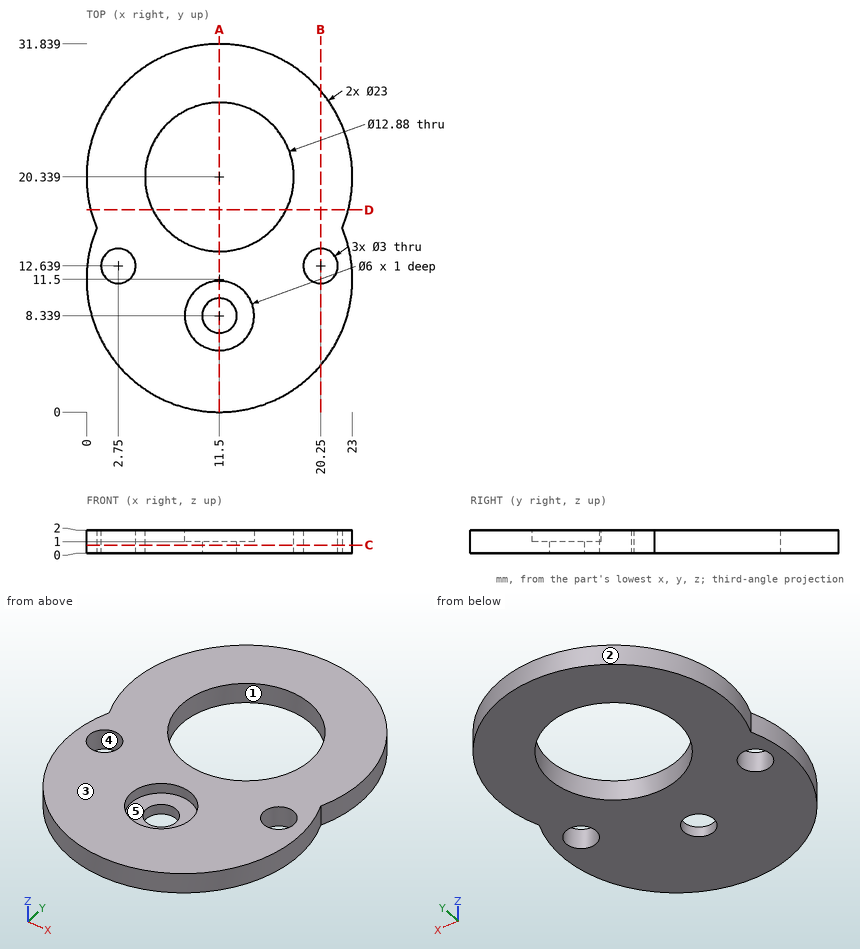
Could you check a few things on this drawing? It's one solid part, dimensions in mm from its lowest x, y, z. A direction names the side the tool comes from. Coordinates: 2 decimals unless noted, no trailing zeros. Order: outer loops, then holes, each group sorted by start corner. A loop starts at its lowest first (then second) coordinate and runs counter-clockwise, first axis right, second up. Notation, with made-up numbers: (50, 59) -> (58, 59) arc R34 ccw to (58, 89) -> close; hole circle Ø6 at (-33, -32.5). An arc over 180 degrees is marked (long way). Answer in a Markdown table with one row per item.
(1) Thinking about a two-plate mould opening in X: for the marked faces 1, 2 and 3, which applies, +X half, -X half, draft (parallel to the pull), parting line (faces both ways), or undercut?
Answer key:
| item | result |
|---|---|
| face 1 | undercut |
| face 2 | parting line |
| face 3 | draft |
(2) Will this pin go through, and if not, where does the flat tip stop? pin 1 Ø1.8 at (x, y) = (10.5, 8) entering from +Z.
Answer key:
| item | result |
|---|---|
| pin 1 | z = 1 |
(3) Please list where these lines run through material, in increasing order: probe 1 along X at (y, z) = (12.5, 1); probe 2 along Y at (x, z) = (11, 0.45) (1 decimal); probe 3 along Y at (x, z) = (20.5, 0.55) (1 decimal).
Answer key:
| item | result |
|---|---|
| probe 1 | 0.04 to 1.26, 4.24 to 18.76, 21.74 to 22.96 |
| probe 2 | 0 to 6.9, 9.8 to 13.9, 26.8 to 31.8 |
| probe 3 | 4.3 to 11.2, 14.1 to 27.5 |
(4) I want a section at B-B on x = 20.25. List the corners of the cut face in (y, z) for me.
Answer key:
| item | result |
|---|---|
| outline | (4.04, 0) -> (11.14, 0) -> (11.14, 2) -> (4.04, 2) -> close; (14.14, 0) -> (27.8, 0) -> (27.8, 2) -> (14.14, 2) -> close |
(5) On a 3-axis mill with a long thin cutter (end or side, diameter ignored), from which of +Z, -Z, +X, -X, +Y, -Y can I reach the whole of each face in a straight line? I mean the marked faces 4 and 5. Say none if no direction works.
Answer key:
| item | result |
|---|---|
| face 4 | +Z, -Z |
| face 5 | +Z |
(6) I want a section at A-A on x = 11.5. List the corners of the cut face in (y, z) for me.
Answer key:
| item | result |
|---|---|
| outline | (0, 0) -> (6.84, 0) -> (6.84, 1) -> (5.34, 1) -> (5.34, 2) -> (0, 2) -> close; (9.84, 0) -> (13.9, 0) -> (13.9, 2) -> (11.34, 2) -> (11.34, 1) -> (9.84, 1) -> close; (26.78, 0) -> (31.84, 0) -> (31.84, 2) -> (26.78, 2) -> close |
(7) I want a section at C-C on z = 0.7. List the corners of the cut face in (x, y) for me, then the cut area to 3 significant figures.
Answer key:
| item | result |
|---|---|
| outline | (0.88, 15.92) arc R11.5 ccw (long way) to (22.12, 15.92) arc R11.5 ccw (long way) to start; hole circle Ø3 at (2.75, 12.64); hole circle Ø12.88 at (11.5, 20.34); hole circle Ø3 at (11.5, 8.34); hole circle Ø3 at (20.25, 12.64) |
| area | 462 mm^2 |
(8) I want a section at D-D on y = 17.5. List the corners of the cut face in (x, z) for me (1 decimal).
Answer key:
| item | result |
|---|---|
| outline | (0.4, 0) -> (5.7, 0) -> (5.7, 2) -> (0.4, 2) -> close; (17.3, 0) -> (22.6, 0) -> (22.6, 2) -> (17.3, 2) -> close |
